Geometry check sheet. Reference: the model listing, model coordinates, mm. A direction names the side the tool comes from. Round coordinates to 2 decimals unless told otherwise and drop trailing zeros. Loops run counter-clockwise (first coordinate to the right, second up) from the corner with the lowest first, then second, coordinate; pieces in that order, holes last. Notation, with made-up numbers: (35.25, 3) - (94.25, 3) arc R8 ccw to (94.25, 8) - close; hole circle Ø5 at (46, 22.5). An arc over 180 degrees is marked (long way). Write item = value, one per line.
```python
from build123d import *

# Parameters (mm, degrees)
BOSS_EXTRUDE1_DEPTH = 5


with BuildPart() as part:
    # Sketch1 → Boss-Extrude1 (new, symmetric)
    with BuildSketch(Plane.XY):
        with BuildLine():
            Line((0, 149.822394855), (-31.25, 95.695807118))
            ThreePointArc((-31.25, 95.695807118), (-22.465390309, 62.911197427), (-55.25, 54.126587737))
            Line((-55.25, 54.126587737), (-86.5, 0))
            Line((-86.5, 0), (-24, 16.746824527))
            ThreePointArc((-24, 16.746824527), (0, 40.746824527), (24, 16.746824527))
            Line((24, 16.746824527), (86.5, 0))
            Line((86.5, 0), (55.25, 54.126587737))
            ThreePointArc((55.25, 54.126587737), (22.465390309, 62.911197427), (31.25, 95.695807118))
            Line((31.25, 95.695807118), (0, 149.822394855))
        make_face()
    extrude(amount=BOSS_EXTRUDE1_DEPTH, both=True)


solid = part.part
```
(1) Section check C-C (x = 43.25). Enter the section's corners in (y, z), then the cut area to 3 significant figures.
Answers follow:
outline = (11.59, -5) - (50.91, -5) - (50.91, 5) - (11.59, 5) - close
area = 393 mm²
(2) Section check B-B (z = -2.25). Enter the section's corners in (x, y).
Answers follow:
outline = (-86.5, 0) - (-24, 16.75) arc R24 cw to (24, 16.75) - (86.5, 0) - (55.25, 54.13) arc R24 cw to (31.25, 95.7) - (0, 149.82) - (-31.25, 95.7) arc R24 cw to (-55.25, 54.13) - close
(3) Set-up check for faces 4 (the flat face through (54.81, 8.49, 0.07)), 5 (the flat face through (71.094, 26.684, 0.07)): record each of +Z, -Z, +X, -X, +Y, -Y from which the full face is reachable in a straight line by a thin tool's end or side.
Answers follow:
face_4 = +Z, -Z, -Y
face_5 = +Z, -Z, +X, +Y
(4) Scan lines: L1, parallel to Y at x = 28.5, z = 0.5; L2, parallel to X at y = 26, z = -0.25; L3, parallel to X at y = 24, z = -0.75. Record each from-to range of solid material in increasing order. Write a range as [from, to].
Answers follow:
L1 = [15.54, 55.98], [93.84, 100.46]
L2 = [-71.49, -22.14], [22.14, 71.49]
L3 = [-72.64, -22.88], [22.88, 72.64]
(5) Mould release check, pull along X, two halves, no side actions. Record for faces 1 (the flat face through (15.844, 122.38, 0.07)), 2 (the flat face through (-70.656, 27.442, 0.07)), 3 (the cylindrical face through (22.734, 62.457, 0.07)): pulls with the +X half, pulls with the -X half, needs draft (parallel to the pull), parting line crosses it, or undercut.
Answers follow:
face_1 = pulls with the +X half
face_2 = pulls with the -X half
face_3 = undercut
(6) Gauge pin test, flat ends, axial feed: pin 1 (1 mm diameter, centred on x = 22, z = 2, fed in from +Y); pin 2 (3 mm diameter, centred on y = 26, z = -2, fed in from -X); pin 3 (5 mm diameter, centred on x = 35.5, z = 2.5, fed in from -Y). Record the tip position at first contact, or that the pin passes through.
Answers follow:
pin_1 = 112.58
pin_2 = -72.35
pin_3 = 13
(7) Section check A-A (y = 35.5). Enter the section's corners in (x, z), then the cut area to 3 significant figures.
Answers follow:
outline = (-66, -5) - (-14.98, -5) - (-14.98, 5) - (-66, 5) - close; (14.98, -5) - (66, -5) - (66, 5) - (14.98, 5) - close
area = 1,020 mm²
(8) Section check D-D (y = 91.5). Enter the section's corners in (x, z), then the cut area to 3 significant figures.
Answers follow:
outline = (-25.91, -5) - (25.91, -5) - (25.91, 5) - (-25.91, 5) - close
area = 518 mm²
